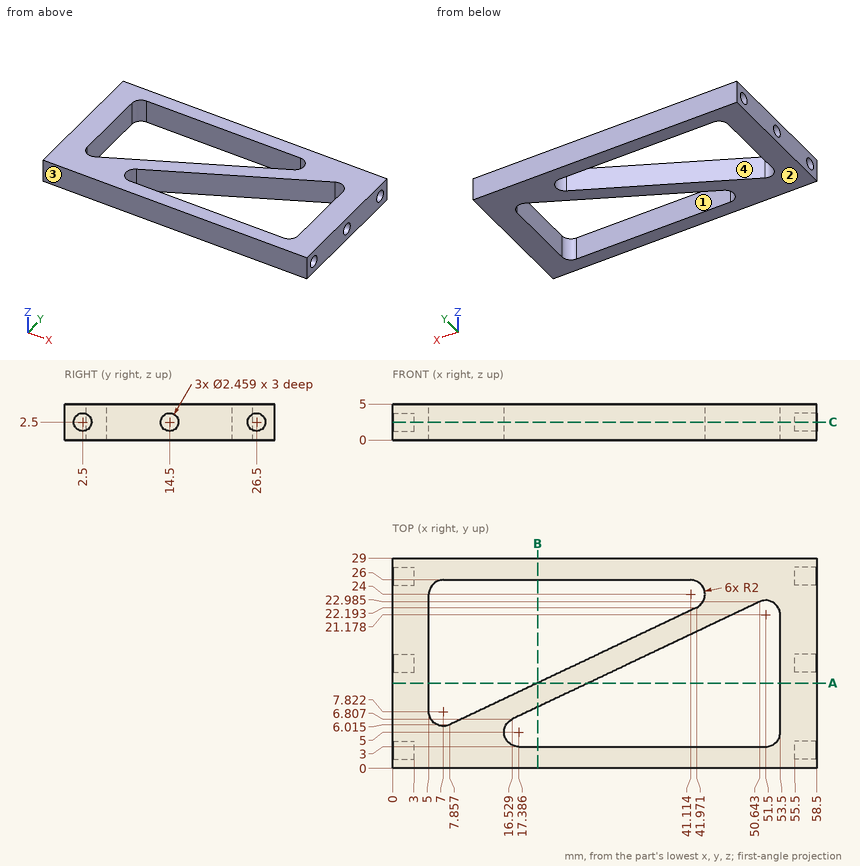
Design review of the part shown in the three views and the two pictorial views. Dimensions are in mm from the part's minimum x, y and z. A direction names the side the tool comes from. Round coordinates to 2 decimals unless told otherwise and drop trailing zeros. Loops run counter-clockwise (first coordinate to the right, second up) from the corner with the lowest first, then second, coordinate; pieces in that order, holes last.
1) The part is to be moulded in two halves that separate along X. For the marked faces 3 and 4, say which applies: pulls with the +X half, pulls with the -X half, needs draft (parallel to the pull), parting line crosses it, or undercut.
Values follow:
face 3: needs draft
face 4: undercut
2) Consider section A-A on y = 11.75. State the section outline as (x, z) points, then the cut area to 3 significant figures.
Values follow:
outline: (0, 0) - (5, 0) - (5, 5) - (0, 5) - close; (19.95, 0) - (26.95, 0) - (26.95, 5) - (19.95, 5) - close; (53.5, 0) - (58.5, 0) - (58.5, 5) - (53.5, 5) - close
area: 85.0 mm2
3) Wall thickness on line 1 along Y through (x, z) = (56.25, 2.5); line 2 along Z through (x, y) = (57.6, 2.5); line 3 along X through (y, z) = (9.25, 0.9): over which ranges is each line inside the solid? List them lowest first.
Values follow:
line 1: y = 0 to 1.27, 3.73 to 13.27, 15.73 to 25.27, 27.73 to 29
line 2: z = 0 to 1.27, 3.73 to 5
line 3: x = 0 to 5, 14.68 to 21.68, 53.5 to 58.5
4) Consider section C-C on z = 2.5. Give the number of separate pieces and of enclosed holes in the cut face, then the cut area to 3 significant figures.
Values follow:
separate pieces: 1
enclosed holes: 2
area: 723 mm2
5) Tool access review of the marked faces 1 and 2: name each direction out of +Z, -Z, +X, -X, +Y, -Y from which nothing blocks a thin tool from reaching the whole face with its end or side.
Values follow:
face 1: +Z, -Z
face 2: -Z, +X, -X, +Y, -Y
6) Clearance check with flat-ended pins moving along their axes: P1, Ø1.5, axis at x = 10.5, y = 10, coming from the +Z side; P2, Ø2, axis at y = 14.5, z = 2.5, coming from the -X side; P3, Ø2, axis at y = 2.5, z = 2.5, coming from the +X side. State where each tip first meets the part, or that it passes through.
Values follow:
P1: passes through
P2: stops at x = 3
P3: stops at x = 55.5
7) Consider section B-B on x = 20. State the section outline as (y, z) points.
Values follow:
outline: (0, 0) - (3, 0) - (3, 5) - (0, 5) - close; (8.45, 0) - (11.77, 0) - (11.77, 5) - (8.45, 5) - close; (26, 0) - (29, 0) - (29, 5) - (26, 5) - close
